Input: part model. Units: mm. Frame: model coordinates. Face numbers are marked on the shaded views. A direction names the side the tool comes from. Give positions to 0.01 mm unless a question says otherwise; leave off trailing zeros. Loops run counter-clockwise (first coordinate to the right, second up) from the corner with the lowest first, then second, coordinate; pieces in that order, holes last. Notation, with made-up numbers: M 15,-16.75 L 36,-16.75 A18 cw 36,-2.75 Z; hole C 13.5,1 d5. An arc over 180 degrees is marked long. Use CSV: the item, a comma, the result in double quotes. Start each with the question number.
Q1. Pull-direction query (Z, two-part tool) for the marked faces 1 and 2; classes: released by +Z, released by -Z, zero draft, split by the parting line, or undercut.
Q2. Material intervals for line 1 along Z through (x, y) = (362.2, -112.6); line 2 along Z through (x, y) = (372.5, -73); line 3 along Y through (x, z) = (363, 142.5), sorted ascending.
Q3. Section A-A, the plane z = 177.65. Output: boundary loops of the cut face in (x, y).
Q4. Section C-C, the plane x = 367.5. State how many separate pieces and enclosed holes the cut face has, plus the area to 3 significant figures.
Q5. Section B-B, the plane z = 230. Output: boundary loops of the cut face in (x, y), plus the area to 3 significant figures.
Q6. Reachability of the marked faces 3, 4 and 5 from +Z, -Z, +X, -X, +Y, -Y: full face, straight path, thin tool, end or side. Return the list, or none.
Q7. Pin query (flat end, axial travel): pin 1 (5 mm diameter, centred on x = 371.5, z = 140.5, fed in from -Y); pin 2 (12 mm diameter, centred on x = 362, y = -65.5, fed in from +Z); pin 3 (1.5 mm diameter, centred on x = 369.5, y = -65, fed in from -Z); pin 4 (4 mm diameter, centred on x = 363, z = 287, fed in from -Y). Return the tip coordinate at first contact, or that it passes through.
Q8. Section D-D, the plane z = 295. Output: boundary loops of the cut face in (x, y), plus the area to 3 significant figures.
from build123d import *

# Parameters (mm, degrees)
CYLINDER044_R                 = 2.2
CYLINDER044_DEPTH             = 26
CYLINDER044_ROLL_ANGLE        = -90
ARRAY011_X_COUNT              = 2
ARRAY011_X_PITCH              = 8
ARRAY011_Z_COUNT              = 2
ARRAY011_Z_PITCH              = 9
BOX034_W                      = 24
BOX034_H                      = 10
BOX034_DEPTH                  = 17
SKETCH030_R                   = 3
PAD030_DEPTH                  = 9
BOX035_W                      = 35
BOX035_H                      = 15
BOX035_DEPTH                  = 20
BOX032_W                      = 23
BOX032_H                      = 3
BOX032_DEPTH                  = 20
SKETCH024_R                   = 3
PAD024_DEPTH                  = 4
SKETCH025_R                   = 3
PAD025_DEPTH                  = 4
BOX029_W                      = 20
BOX029_H                      = 17
BOX029_DEPTH                  = 10
FILLET009_R                   = 1
FILLET009_ROLL_ANGLE          = 90
FILLET010_1_R                 = 2
FILLET010_2_R                 = 1
BOX028_W                      = 167
BOX028_H                      = 10
BOX028_DEPTH                  = 17
CYLINDER040_R                 = 2.2
CYLINDER040_DEPTH             = 18
CYLINDER040_ROLL_ANGLE        = -90
ARRAY008_X_COUNT              = 2
ARRAY008_X_PITCH              = 49.2
ARRAY008_Z_COUNT              = 2
ARRAY008_Z_PITCH              = 10.3
PAD029_DEPTH                  = 6
PAD028_DEPTH                  = 10
CHAMFER003_SIZE               = 3
PART_MIRRORING005_PITCH_ANGLE = 90


with BuildPart() as obj1:
    # Cylinder044 → Cylinder044 (new body)
    with BuildSketch(Plane.XY):
        Circle(CYLINDER044_R)
    extrude(amount=CYLINDER044_DEPTH)


with BuildPart() as obj1_1:
    # Cylinder044 roll: moved
    add(obj1.part.rotate(Axis((0, 0, 0), (1, 0, 0)), CYLINDER044_ROLL_ANGLE))


with BuildPart() as obj1_2:
    # Cylinder044 placement: moved
    add(obj1_1.part.moved(Location((202, 0, 4))))

    # Array011 X: obj1_2


with BuildPart() as obj1_3:
    add(obj1_2.part)
    with Locations(*[(i * ARRAY011_X_PITCH, 0, 0) for i in range(1, ARRAY011_X_COUNT)]):
        add(obj1_2.part)

    # Array011 Z: obj1_2


with BuildPart() as obj1_4:
    add(obj1_3.part)
    with Locations(*[(0, 0, i * ARRAY011_Z_PITCH) for i in range(1, ARRAY011_Z_COUNT)]):
        add(obj1_3.part)


with BuildPart() as obj1_5:
    # Array011 placement: moved
    add(obj1_4.part.moved(Location((-171, -5, 0))))


with BuildPart() as obj2:
    # Box034 → Box034 (new body)
    with BuildSketch(Plane(origin=(26, 6, 0), x_dir=(1, 0, 0), z_dir=(0, 0, 1))):
        with Locations((12, 5)):
            Rectangle(BOX034_W, BOX034_H)
    extrude(amount=BOX034_DEPTH)


with BuildPart() as obj3:
    # Sketch030 → Pad030 (new body)
    with BuildSketch(Plane(origin=(50, 6, 0), x_dir=(1, 0, 0), z_dir=(0, -1, 0))):
        with BuildLine():
            Line((0, 17), (-36, 17))
            ThreePointArc((-36, 17), (-44.500015, 8.5), (-36, 0))
            Line((-36, 0), (0, 0))
            Line((0, 0), (0, 17))
        make_face()
        with Locations((-36.000015, 8.5)):
            Circle(SKETCH030_R, mode=Mode.SUBTRACT)
    extrude(amount=PAD030_DEPTH)


with BuildPart() as obj4:
    # Box035 → Box035 (new body)
    with BuildSketch(Plane(origin=(-2, -5, 0), x_dir=(1, 0, 0), z_dir=(0, 0, 1))):
        with Locations((17.5, 7.5)):
            Rectangle(BOX035_W, BOX035_H)
    extrude(amount=BOX035_DEPTH)


with BuildPart() as obj5:
    # Box032 → Box032 (new body)
    with BuildSketch(Plane(origin=(80.5, 1, 0), x_dir=(1, 0, 0), z_dir=(0, 0, 1))):
        with Locations((11.5, 1.5)):
            Rectangle(BOX032_W, BOX032_H)
    extrude(amount=BOX032_DEPTH)


with BuildPart() as obj6:
    # Sketch024 → Pad024 (new body)
    with BuildSketch(Plane.XY):
        with BuildLine():
            Line((0, 17), (20, 17))
            ThreePointArc((20, 0), (28.500019, 8.5), (20, 17))
            Line((20, 0), (0, 0))
            Line((0, 0), (0, 17))
        make_face()
        with Locations((20.000019, 8.5)):
            Circle(SKETCH024_R, mode=Mode.SUBTRACT)
    extrude(amount=PAD024_DEPTH)


with BuildPart() as obj7:
    # Sketch025 → Pad025 (new body)
    with BuildSketch(Plane.XY.offset(14)):
        with BuildLine():
            Line((0, 17), (20, 17))
            ThreePointArc((20, 0), (28.500019, 8.5), (20, 17))
            Line((20, 0), (0, 0))
            Line((0, 0), (0, 17))
        make_face()
        with Locations((20.000019, 8.5)):
            Circle(SKETCH025_R, mode=Mode.SUBTRACT)
    extrude(amount=PAD025_DEPTH)


with BuildPart() as obj8:
    # Box029 → Box029 (new body)
    with BuildSketch(Plane(origin=(-16, 0, 4), x_dir=(1, 0, 0), z_dir=(0, 0, 1))):
        with Locations((10, 8.5)):
            Rectangle(BOX029_W, BOX029_H)
    extrude(amount=BOX029_DEPTH)

    # Fusion009003028: union obj6, obj7
    add(obj6.part)
    add(obj7.part)

    # Fillet009
    fillet009_edges = [obj8.edges().sort_by_distance(p)[0] for p in [
        (0, 8.5, 18),
        (-16, 0, 9),
        (-16, 17, 9),
        (0, 8.5, 0),
    ]]
    fillet(fillet009_edges, radius=FILLET009_R)


with BuildPart() as obj8_1:
    # Fillet009 roll: moved
    add(obj8.part.rotate(Axis((0, 0, 0), (1, 0, 0)), FILLET009_ROLL_ANGLE))


with BuildPart() as obj8_2:
    # Fillet009 placement: moved
    add(obj8_1.part.moved(Location((16, 15, 0))))

    # Fillet010 1
    fillet010_1_edges = [obj8_2.edges().sort_by_distance(p)[0] for p in [
        (16, 1, 8.5),
        (16, 11, 8.5),
    ]]
    fillet(fillet010_1_edges, radius=FILLET010_1_R)

    # Fillet010 2
    fillet010_2_edges = [obj8_2.edges().sort_by_distance(p)[0] for p in [
        (20, 1, 8.5),
        (20, 11, 8.5),
    ]]
    fillet(fillet010_2_edges, radius=FILLET010_2_R)


with BuildPart() as obj8_3:
    # Fillet010 placement: moved
    add(obj8_2.part.moved(Location((149, 0, 0))))


with BuildPart() as obj9:
    # Box028 → Box028 (new body)
    with BuildSketch(Plane(origin=(0, -3, 0), x_dir=(1, 0, 0), z_dir=(0, 0, 1))):
        with Locations((83.5, 5)):
            Rectangle(BOX028_W, BOX028_H)
    extrude(amount=BOX028_DEPTH)

    # Fusion009003029: union obj8
    add(obj8_3.part)

    # Cut023: cut obj5
    add(obj5.part, mode=Mode.SUBTRACT)


with BuildPart() as obj10:
    # Cylinder040 → Cylinder040 (new body)
    with BuildSketch(Plane.XY):
        Circle(CYLINDER040_R)
    extrude(amount=CYLINDER040_DEPTH)


with BuildPart() as obj10_1:
    # Cylinder040 roll: moved
    add(obj10.part.rotate(Axis((0, 0, 0), (1, 0, 0)), CYLINDER040_ROLL_ANGLE))


with BuildPart() as obj10_2:
    # Cylinder040 placement: moved
    add(obj10_1.part.moved(Location((150.075, 41, 13.5))))

    # Array008 X: obj10_2


with BuildPart() as obj10_3:
    add(obj10_2.part)
    with Locations(*[(i * ARRAY008_X_PITCH, 0, 0) for i in range(1, ARRAY008_X_COUNT)]):
        add(obj10_2.part)

    # Array008 Z: obj10_2


with BuildPart() as obj10_4:
    add(obj10_3.part)
    with Locations(*[(0, 0, -i * ARRAY008_Z_PITCH) for i in range(1, ARRAY008_Z_COUNT)]):
        add(obj10_3.part)


with BuildPart() as obj11:
    # Sketch029 → Pad029 (new body)
    with BuildSketch(Plane(origin=(10, 54.8, 0), x_dir=(1, 0, 0), z_dir=(0, -1, 0))):
        Polygon((0, 18.5), (0, 24.5), (50.5, 24.5), (50.5, 0), (40.5, 0), (40.5, 18.5), align=None)
    extrude(amount=PAD029_DEPTH)


with BuildPart() as obj12:
    # Sketch028 → Pad028 (new body)
    with BuildSketch(Plane.YZ):
        Polygon((14, 0), (0, 0), (0, 24.5), (54.8, 24.5), (54.8, 0), (48.8, 0), (48.8, 18.5), (14, 18.5), align=None)
    extrude(amount=PAD028_DEPTH)

    # Fusion009003033: union obj11
    add(obj11.part)


with BuildPart() as obj12_1:
    # Fusion009003033 placement: moved
    add(obj12.part.moved(Location((144.425, -3, 0))))

    # Cut022: cut obj10
    add(obj10_4.part, mode=Mode.SUBTRACT)


with BuildPart() as obj12_2:
    # Cut022 placement: moved
    add(obj12_1.part.moved(Location((-1.725, 0, 0))))

    # Fusion009003034: union obj9
    add(obj9.part)

    # Chamfer003
    chamfer003_edges = [obj12_2.edges().sort_by_distance(p)[0] for p in [
        (142.7, 7, 8.5),
    ]]
    chamfer(chamfer003_edges, length=CHAMFER003_SIZE)

    # Cut027: cut obj4
    add(obj4.part, mode=Mode.SUBTRACT)

    # Fusion009003036: union obj3
    add(obj3.part)

    # Fusion009003037: union obj2
    add(obj2.part)

    # Cut028: cut obj1
    add(obj1_5.part, mode=Mode.SUBTRACT)


with BuildPart() as part_mirroring005:
    # Part__Mirroring005: instance of obj12
    add(obj12_2.part.mirror(Plane(origin=(0, 0, 0), x_dir=(1, 0, 0), z_dir=(0, 1, 0))))


with BuildPart() as part_mirroring005_1:
    # Part__Mirroring005 pitch: moved
    add(part_mirroring005.part.rotate(Axis((0, 0, 0), (0, 1, 0)), PART_MIRRORING005_PITCH_ANGLE))


with BuildPart() as part_mirroring005_2:
    # Part__Mirroring005 placement: moved
    add(part_mirroring005_1.part.moved(Location((359, -63, 326))))


solid = part_mirroring005_2.part
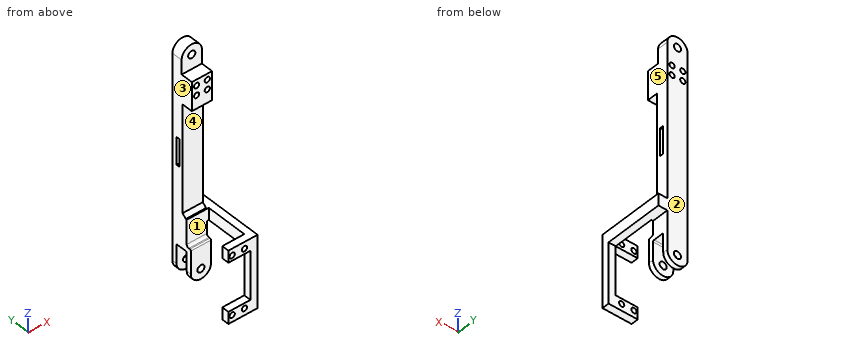
A:
1,face 1,"undercut"
1,face 2,"zero draft"
2,line 1,"122.8 to 126.25, 130.65 to 132.8, 173.3 to 175.45, 179.85 to 183.3"
2,line 2,"157 to 183.3, 276 to 284.86, 289.14 to 292.86, 297.14 to 300"
2,line 3,"-78 to -74, -64 to -60"
3,outline,"M 359,-114.8 L 360,-114.8 L 360,-108.8 L 359,-108.8 Z; M 359,-74 L 377.5,-74 L 377.5,-108.8 L 374.7,-108.8 L 374.7,-114.8 L 383.5,-114.8 L 383.5,-60 L 359,-60 Z; M 364.4,-114.8 L 370.3,-114.8 L 370.3,-108.8 L 364.4,-108.8 Z"
4,separate pieces,"6"
4,enclosed holes,"1"
4,area,"2,100 mm^2"
5,outline,"M 359,-70 L 376,-70 L 376,-67 L 359,-67 Z; M 359,-64 L 376,-64 L 376,-60 L 359,-60 Z"
5,area,"119 mm^2"
6,face 3,"+Z, -Z, -X, +Y, -Y"
6,face 4,"+X, -X, -Y"
6,face 5,"+Z, +X, +Y, -Y"
7,pin 1,"y = -78"
7,pin 2,"z = 320.5"
7,pin 3,"z = 156.66"
7,pin 4,"through"
8,outline,"M 359,-79 L 360.8,-79 L 360.8,-60 L 359,-60 Z; M 365.2,-79 L 369.8,-79 L 369.8,-60 L 365.2,-60 Z; M 374.2,-79 L 376,-79 L 376,-60 L 374.2,-60 Z"
8,area,"156 mm^2"
